The listing builds one solid part. Answer for the finished solid, in the listing's coordinates (mm). A direction names the side the tool comes from. Coordinates: 2 decimals unless noted, no trailing zeros. Order: outer loops, then holes, each group sorted by start corner. A loop starts at its lowest first (then second) coordinate and runs counter-clockwise, first axis right, second up.
from build123d import *

# Parameters (mm, degrees)
CROQUIS1_R                 = 3
SALIENTE_EXTRUIR2_DEPTH    = 20
CROQUIS2_R                 = 1.5
CORTAR_EXTRUIR1_DEPTH      = 4
CORTAR_EXTRUIR1_DEPTH_BACK = 4
REDONDEO7_R                = 1


with BuildPart() as part:
    # Croquis1 → Saliente-Extruir2 (new body)
    with BuildSketch(Plane.XY):
        Circle(CROQUIS1_R)
    extrude(amount=SALIENTE_EXTRUIR2_DEPTH)

    # Croquis2 → Cortar-Extruir1 (cut, two sides)
    with BuildSketch(Plane(origin=(0, 0, 0), x_dir=(1, 0, 0), z_dir=(0, 1, 0))) as cortar_extruir1_sk:
        with Locations((0, -10)):
            Circle(CROQUIS2_R)
        Polygon((-3, -20), (0, -16), (3, -20), align=None)
    extrude(amount=CORTAR_EXTRUIR1_DEPTH, mode=Mode.SUBTRACT)
    extrude(cortar_extruir1_sk.sketch, amount=-CORTAR_EXTRUIR1_DEPTH_BACK, mode=Mode.SUBTRACT)

    # Redondeo7
    redondeo7_edges = [part.edges().sort_by_distance(p)[0] for p in [
        (-3, 0, 0),
        (0, 0, 16),
    ]]
    fillet(redondeo7_edges, radius=REDONDEO7_R)


solid = part.part
1) Each of these flat-tipped pins is pushed along its axis until it touches: P1, Ø2, axis at y = -1.5, z = 7.5, coming from the -X side; P2, Ø2, axis at x = -2.5, z = 7.5, coming from the -Y side; P3, Ø1, axis at x = -2, z = 9.5, coming from the +Y side. Where does it stop, or does it pass through?
2) A tool of negligible diameter and unlimited length cuts with its end or side. For faces 1 (the face through (0, 0, 0)), 2 (the face through (-1.671, 0.04, 18.228)), from which of +Z, -Z, +X, -X, +Y, -Y can it reach the whole face along a straight path? Write none if from no direction.
3) Section B-B (z = 4) is taken. Give the vertices of the cut face in (x, y).
4) Section D-D (z = 18) is taken. Give the vertices of the cut face in (x, y), then the cut area to 3 significant figures.
5) Section A-A (x = 0) is taken. Give the vertices of the cut face in (y, z).
6) Section C-C (z = 10.75) is taken. Give the vertices of the cut face in (x, y), then the cut area to 3 significant figures.
7) Consider L1, parallel to Z at x = 0, y = -1.45; L2, parallel to Z at x = 0.25, y = 2.5; L3, parallel to X at y = 1.75, z = 17.5 (3 decimals). Determine where each line is inside the solid, lowest interval first.
Filled sheet:
1. P1: stops at x = -2.96
1. P2: stops at y = -2.6
1. P3: stops at y = 2.6
2. face 1: -Z, +X, -X, +Y, -Y
2. face 2: +Z, +Y, -Y
3. outline: circle Ø6 at (0, 0)
4. outline: (-1.5, -2.6) - (-1.5, 2.6) arc R3 ccw to start; (1.5, -2.6) arc R3 ccw to (1.5, 2.6) - close
4. area: 11.1 mm2
5. outline: (-3, 1) arc R1 ccw to (-2, 0) - (2, 0) arc R1 ccw to (3, 1) - (3, 8.5) - (-3, 8.5) - close; (-3, 11.5) - (3, 11.5) - (3, 16.67) - (-3, 16.67) - close
6. outline: (-1.3, -2.7) - (-1.3, 2.7) arc R3 ccw to start; (1.3, -2.7) arc R3 ccw to (1.3, 2.7) - close
6. area: 13.2 mm2
7. L1: z = 0 to 8.5, 11.5 to 16.67
7. L2: z = 0.14 to 8.52, 11.48 to 16.7
7. L3: x = -2.437 to -1.125, 1.125 to 2.437
